Can you work these out from the model? Positions are in its coordinate system, mm. Round coordinates to 2 decimals unless told otherwise and drop trailing zeros. Loops run counter-clockwise (first coordinate to the right, second up) from the corner with the lowest first, then second, coordinate; pieces in that order, holes last. Notation, with made-up numbers: M -27.75,59 L 25.25,59 A12 ccw 25.25,80 Z; hole C 38,35.25 d6. An arc over 180 degrees is marked long. Return JSON: item names as keys, results as strings.
```python
from build123d import *

# Parameters (mm, degrees)
BOSS_EXTRUDE1_DEPTH = 200


with BuildPart() as part:
    # Sketch1 → Boss-Extrude1 (new body)
    with BuildSketch(Plane(origin=(0, 0, 0), x_dir=(1, 0, 0), z_dir=(0, 1, 0))):
        with BuildLine():
            Line((-3.239339866, -2.878050905), (-3.239339866, -5.427441221))
            ThreePointArc((-3.239339866, -5.427441221), (-2.961547411, -5.843187011), (-2.471141815, -5.745639273))
            Line((-2.471141815, -5.745639273), (-0.25, -3.524497458))
            Line((-0.25, -3.524497458), (-0.25, 3.524497458))
            Line((-0.25, 3.524497458), (-2.471141814, 5.745639272))
            ThreePointArc((-2.471141814, 5.745639272), (-2.961547408, 5.84318701), (-3.239339864, 5.427441222))
            Line((-3.239339864, 5.427441222), (-3.239339864, 2.878050849))
            Line((-3.239339864, 2.878050849), (-4.939339838, 2.878050849))
            Line((-4.939339838, 2.878050849), (-5.189339838, 2.878050849))
            Line((-5.189339838, 2.878050849), (-5.189339838, -2.878050905))
            Line((-5.189339838, -2.878050905), (-3.239339866, -2.878050905))
        make_face()
    extrude(amount=BOSS_EXTRUDE1_DEPTH)


solid = part.part
```
Q1. I'm going to push flat-ended pins straight in: pin 1 Ø1 at (x, y) = (-4.5, 116) entering from +Z; pin 2 Ø0.8 at (y, z) = (141.5, 4.5) entering from -X; pin 3 Ø3 at (y, z) = (138.5, -4) entering from -X. Where does each tip first touch, or does it pass through?
Results:
{"pin 1": "stops at z = 2.88", "pin 2": "stops at x = -3.24", "pin 3": "stops at x = -5.19"}
Q2. If I drill on line 1 along Z through (x, y) = (-4.45, 13.5); line 2 along X through (y, z) = (94, -3); line 3 along Z through (x, y) = (-2.7, 30.5), over which ranges is the centre line in solid material (lowest first)?
Results:
{"line 1": "z = -2.88 to 2.88", "line 2": "x = -3.24 to -0.25", "line 3": "z = -5.87 to 5.87"}
Q3. Suppose I cut it at A-A, the plane y = 125.5. Please give me the cut outline in (x, z).
Results:
{"outline": "M -5.19,-2.88 L -3.24,-2.88 L -3.24,-5.43 A0.45 ccw -2.47,-5.75 L -0.25,-3.52 L -0.25,3.52 L -2.47,5.75 A0.45 ccw -3.24,5.43 L -3.24,2.88 L -5.19,2.88 Z"}
Q4. Suppose I cut it at B-B, the plane x = -4.05. Please give me the cut outline in (y, z), plus the area to 3 significant figures.
Results:
{"outline": "M 0,-2.88 L 200,-2.88 L 200,2.88 L 0,2.88 Z", "area": "1,150 mm2"}
